```python
from build123d import *

# Parameters (mm, degrees)
SKETCH1_W                    = 155
SKETCH1_H                    = 180
BASE_FLANGE1_DEPTH           = 0.5
EDGE_FLANGE1_STRIP_W         = 3
EDGE_FLANGE1_STRIP_H         = 0.5
EDGE_FLANGE1_STRIP_CUT_DEPTH = 180
EDGE_FLANGE1_DEPTH           = 180
EDGE_FLANGE3_STRIP_CUT_DEPTH = 154.5
EDGE_FLANGE3_DEPTH           = 154.5
EDGE_FLANGE4_DEPTH           = 154.5
SKETCH25_W                   = 0.5
SKETCH25_H                   = 41.5
BOSS_EXTRUDE1_DEPTH          = 7
CUT_EXTRUDE2_DEPTH           = 0.5
EDGE_FLANGE5_STRIP_CUT_DEPTH = 154.5
EDGE_FLANGE5_DEPTH           = 154.5
EDGE_FLANGE6_STRIP_CUT_DEPTH = 154.5
EDGE_FLANGE6_DEPTH           = 154.5
SKETCH41_W                   = 0.5
SKETCH41_H                   = 41.5
BOSS_EXTRUDE2_DEPTH          = 7
CUT_EXTRUDE3_DEPTH           = 0.5
SKETCH45_R                   = 11
SKETCH45_R_2                 = 12
CUT_EXTRUDE6_DEPTH           = 2
SKETCH51_R                   = 1.5
CUT_EXTRUDE7_DEPTH           = 2


# Sheet-metal steps are written as plain solids
with BuildPart() as part:
    # Sketch1 → Base-Flange1 (new body)
    with BuildSketch(Plane(origin=(0, 0, 0), x_dir=(1, 0, 0), z_dir=(0, 1, 0))):
        with Locations((77.5, -90)):
            Rectangle(SKETCH1_W, SKETCH1_H)
    extrude(amount=-BASE_FLANGE1_DEPTH)

    # Edge-Flange1 strip (across the edge) → Edge-Flange1 strip cut (cut)
    with BuildSketch(Plane.XY):
        with Locations((-1, -0.25)):
            Rectangle(EDGE_FLANGE1_STRIP_W, EDGE_FLANGE1_STRIP_H)
    extrude(amount=EDGE_FLANGE1_STRIP_CUT_DEPTH, mode=Mode.SUBTRACT)

    # Edge-Flange1 section (across the edge) → Edge-Flange1 (add)
    with BuildSketch(Plane.XY):
        with BuildLine():
            Line((-0.5, 0.5), (-0.5, 42))
            Line((-0.5, 42), (0, 42))
            Line((0, 42), (0, 0.5))
            ThreePointArc((0, 0.5), (0.146446609, 0.146446609), (0.5, 0))
            Line((0.5, 0), (0.5, -0.5))
            ThreePointArc((0.5, -0.5), (-0.207106781, -0.207106781), (-0.5, 0.5))
        make_face()
    extrude(amount=EDGE_FLANGE1_DEPTH)

    # Edge-Flange3 strip (across the edge) → Edge-Flange3 strip cut (cut)
    with BuildSketch(Plane(origin=(155, 0, 0), x_dir=(0, 0.7071067811865512, 0.7071067811865438), z_dir=(-1, 0, 0))):
        Polygon((-2.328427125, 1.621320344), (-0.207106781, -0.5), (0.146446609, -0.146446609), (-1.974873734, 1.974873734), align=None)
    extrude(amount=EDGE_FLANGE3_STRIP_CUT_DEPTH, mode=Mode.SUBTRACT)

    # Edge-Flange3 section (across the edge) → Edge-Flange3 (add)
    with BuildSketch(Plane(origin=(155, 0, 0), x_dir=(0, 0.7071067811865512, 0.7071067811865438), z_dir=(-1, 0, 0))):
        with BuildLine():
            Line((-0.5, 0.207106781), (-0.5, 10))
            Line((-0.5, 10), (0, 10))
            Line((0, 10), (0, 0.207106781))
            ThreePointArc((0, 0.207106781), (0.038060234, 0.015765065), (0.146446609, -0.146446609))
            Line((0.146446609, -0.146446609), (-0.207106781, -0.5))
            ThreePointArc((-0.207106781, -0.5), (-0.423879533, -0.175576651), (-0.5, 0.207106781))
        make_face()
    extrude(amount=EDGE_FLANGE3_DEPTH)

    # Edge-Flange4 section (across the edge) → Edge-Flange4 (add)
    with BuildSketch(Plane(origin=(155, 7.363961031, -7.363961031), x_dir=(0, 0, 1), z_dir=(-1, 0, 0))):
        with BuildLine():
            Line((-0.5, 0.414213562), (-0.5, 34.636038969))
            Line((-0.5, 34.636038969), (0, 34.636038969))
            Line((0, 34.636038969), (0, 0.414213562))
            ThreePointArc((0, 0.414213562), (0.076120467, 0.03153013), (0.292893219, -0.292893219))
            Line((0.292893219, -0.292893219), (-0.060660172, -0.646446609))
            ThreePointArc((-0.060660172, -0.646446609), (-0.385819299, -0.159811586), (-0.5, 0.414213562))
        make_face()
    extrude(amount=EDGE_FLANGE4_DEPTH)

    # Sketch25 → Boss-Extrude1 (add)
    with BuildSketch(Plane(origin=(0, 0, 0), x_dir=(-1, 0, 0), z_dir=(0, 0, -1))):
        with Locations((0.25, 21.25)):
            Rectangle(SKETCH25_W, SKETCH25_H)
    extrude(amount=BOSS_EXTRUDE1_DEPTH)

    # Sketch28 → Cut-Extrude2 (cut)
    with BuildSketch(Plane.ZY.offset(0.5)):
        Polygon((-7.360561455, 7.860561455), (0, 0.5), (-7.360561455, 0.5), align=None)
    extrude(amount=-CUT_EXTRUDE2_DEPTH, mode=Mode.SUBTRACT)

    # Edge-Flange5 strip (across the edge) → Edge-Flange5 strip cut (cut)
    with BuildSketch(Plane(origin=(0.5, 0, 180), x_dir=(0, 0.7071067811865512, -0.7071067811865438), z_dir=(1, 0, 0))):
        Polygon((-2.328427125, 1.621320344), (-0.207106781, -0.5), (0.146446609, -0.146446609), (-1.974873734, 1.974873734), align=None)
    extrude(amount=EDGE_FLANGE5_STRIP_CUT_DEPTH, mode=Mode.SUBTRACT)

    # Edge-Flange5 section (across the edge) → Edge-Flange5 (add)
    with BuildSketch(Plane(origin=(0.5, 0, 180), x_dir=(0, 0.7071067811865512, -0.7071067811865438), z_dir=(1, 0, 0))):
        with BuildLine():
            Line((-0.5, 0.207106781), (-0.5, 10))
            Line((-0.5, 10), (0, 10))
            Line((0, 10), (0, 0.207106781))
            ThreePointArc((0, 0.207106781), (0.038060234, 0.015765065), (0.146446609, -0.146446609))
            Line((0.146446609, -0.146446609), (-0.207106781, -0.5))
            ThreePointArc((-0.207106781, -0.5), (-0.423879533, -0.175576651), (-0.5, 0.207106781))
        make_face()
    extrude(amount=EDGE_FLANGE5_DEPTH)

    # Edge-Flange6 strip (across the edge) → Edge-Flange6 strip cut (cut)
    with BuildSketch(Plane(origin=(0.5, 7.071067812, 187.071067812), x_dir=(0, 0, -1), z_dir=(1, 0, 0))):
        Polygon((-2.328427125, 1.621320344), (-0.207106781, -0.5), (0.146446609, -0.146446609), (-1.974873734, 1.974873734), align=None)
    extrude(amount=EDGE_FLANGE6_STRIP_CUT_DEPTH, mode=Mode.SUBTRACT)

    # Edge-Flange6 section (across the edge) → Edge-Flange6 (add)
    with BuildSketch(Plane(origin=(0.5, 7.071067812, 187.071067812), x_dir=(0, 0, -1), z_dir=(1, 0, 0))):
        with BuildLine():
            Line((-0.5, 0.207106781), (-0.5, 34.928932188))
            Line((-0.5, 34.928932188), (0, 34.928932188))
            Line((0, 34.928932188), (0, 0.207106781))
            ThreePointArc((0, 0.207106781), (0.038060234, 0.015765065), (0.146446609, -0.146446609))
            Line((0.146446609, -0.146446609), (-0.207106781, -0.5))
            ThreePointArc((-0.207106781, -0.5), (-0.423879533, -0.175576651), (-0.5, 0.207106781))
        make_face()
    extrude(amount=EDGE_FLANGE6_DEPTH)

    # Sketch41 → Boss-Extrude2 (add)
    with BuildSketch(Plane.XY.offset(180)):
        with Locations((-0.25, 21.25)):
            Rectangle(SKETCH41_W, SKETCH41_H)
    extrude(amount=BOSS_EXTRUDE2_DEPTH)

    # Sketch44 → Cut-Extrude3 (cut)
    with BuildSketch(Plane.ZY.offset(0.5)):
        Polygon((180, 0.5), (187, 7.5), (187, 0.5), align=None)
    extrude(amount=-CUT_EXTRUDE3_DEPTH, mode=Mode.SUBTRACT)

    # Sketch45 → Cut-Extrude6 (cut)
    with BuildSketch(Plane.ZY.offset(0.5)):
        with Locations(Location((16.636038969, 21, 0), (0, 0, 270))):
            Circle(SKETCH45_R)
        with Locations(Location((163.071067812, 21, 0), (0, 0, 270))):
            Circle(SKETCH45_R_2)
    extrude(amount=-CUT_EXTRUDE6_DEPTH, mode=Mode.SUBTRACT)

    # Sketch51 → Cut-Extrude7 (cut)
    with BuildSketch(Plane.ZY.offset(0.5)):
        with Locations(Location((16.636038969, 38, 0), (0, 0, 270))):
            Circle(SKETCH51_R)
        with Locations(Location((33.636038969, 21, 0), (0, 0, 270))):
            Circle(SKETCH51_R)
        with Locations(Location((16.636038969, 4, 0), (0, 0, 270))):
            Circle(SKETCH51_R)
        with Locations(Location((-0.363961031, 21, 0), (0, 0, 270))):
            Circle(SKETCH51_R)
    extrude(amount=-CUT_EXTRUDE7_DEPTH, mode=Mode.SUBTRACT)


solid = part.part
```
The model under review builds one solid part; all positions refer to its coordinate system, in mm. A direction names the side the tool comes from. Give positions to 0.01 mm unless a question says otherwise; leave off trailing zeros. Loops run counter-clockwise (first coordinate to the right, second up) from the corner with the lowest first, then second, coordinate; pieces in that order, holes last. Notation, with made-up numbers: (-3, 46.25) - (32, 46.25) arc R32 cw to (32, 81.25) - close; hole circle Ø2 at (67.25, 31.25). An arc over 180 degrees is marked (long way). Answer as a JSON object with one key per item and string values.
Q1. Mouldability with a two-part tool opening along Z and no side actions: class faces 4 (the flat face through (-0.3, 4, 183.5)), 5 (the cylindrical face through (-0.254, 15.086, 25.911)), 6 (the flat face through (0, 21, 89)) as +Z half, -Z half, draft (parallel to the pull), parting line (faces both ways), or undercut.
Worked out:
{"face 4": "+Z half", "face 5": "undercut", "face 6": "draft"}
Q2. Add section A-A on y = 26. State the section outline as (x, z) points.
Worked out:
{"outline": "(-0.5, -7) - (0, -7) - (0, 6.84) - (-0.5, 6.84) - close; (-0.5, 26.43) - (0, 26.43) - (0, 152.16) - (-0.5, 152.16) - close; (-0.5, 173.98) - (0, 173.98) - (0, 187) - (-0.5, 187) - close; (0.5, -7.86) - (155, -7.86) - (155, -7.36) - (0.5, -7.36) - close; (0.5, 187.07) - (155, 187.07) - (155, 187.57) - (0.5, 187.57) - close"}
Q3. Insertion check: pin 1 (12 mm diameter, centred on y = 8.5, z = 166.5, fed in from +X); pin 2 (0.6 mm diameter, centred on x = -0.5, y = 32, fed in from +Z); pin 3 (0.5 mm diameter, centred on x = 0, y = 0, fed in from +Z). Each pin has a flat end and moves straight along its axis. Give the tip position at first contact, or say it passes through.
Worked out:
{"pin 1": "stops at x = 0", "pin 2": "stops at z = 187", "pin 3": "stops at z = 180"}
Q4. Add section B-B on x = 79.5. State the section outline as (y, z) points, plus the area to 3 significant figures.
Worked out:
{"outline": "(-0.5, 0.21) arc R1 ccw to (-0.21, -0.5) - (6.72, -7.42) arc R1.5 ccw to (7.78, -7.86) - (42, -7.86) - (42, -7.36) - (7.78, -7.36) arc R1 cw to (7.07, -7.07) - (0.15, -0.15) arc R0.5 cw to (0, 0.21) - (0, 179.79) arc R0.5 cw to (0.15, 180.15) - (6.92, 186.92) arc R0.5 cw to (7.28, 187.07) - (42, 187.07) - (42, 187.57) - (7.28, 187.57) arc R1 ccw to (6.57, 187.28) - (-0.21, 180.5) arc R1 ccw to (-0.5, 179.79) - close", "area": "135 mm^2"}
Q5. To check wall thickness, follow line 1 along Z through (x, y) = (-0.25, 21); line 2 along Z through (x, y) = (126, 8); line 3 along X through (y, z) = (39.5, 39.5). State the ranges of each line that lie inside material, in increasing order.
Worked out:
{"line 1": "z = -7 to -1.86, 1.14 to 5.64, 27.64 to 32.14, 35.14 to 151.07, 175.07 to 187", "line 2": "z = -7.86 to -7.36, 187.07 to 187.57", "line 3": "x = -0.5 to 0"}
Q6. For faces 1 (the flat face through (77, 0, 89)), 2 (the flat face through (79, 4, -4)), 3 (the flat face through (79, 25, -7.864)), list the 3-axis set-ups (+Z, -Z, +X, -X, +Y, -Y) from which the entire face can be reached by the end or side of a thin tool; tool diameter is ignored.
Worked out:
{"face 1": "+X, +Y", "face 2": "+X, -X, +Y", "face 3": "-Z, +X, -X, +Y, -Y"}
